Could you check a few things on this model? Use its own coordinates, in mm. A direction names the side the tool comes from. Round coordinates to 2 decimals unless told otherwise and drop trailing zeros. Write each loop counter-clockwise with the first axis right and the second up, starting at its lowest first coordinate (ties: lowest second). Pieces come first, ordered by that corner, then holes. Notation, with made-up numbers: (-0.75, -6) -> (31.25, -6) arc R13 ccw to (31.25, 18) -> close; hole circle Ø7 at (-17.75, -13). An arc over 180 degrees is marked (long way). One line per question, with ' | ' between items. Start each with the question number.
1. For faces 1 (the flat face through (-22.662, -5, 23)), 2 (the flat face through (4, 0, 1)), 3 (the flat face through (-17.224, -4.93, 22.376)), which set-ups out of +Z, -Z, +X, -X, +Y, -Y let a thin tool reach every point of the face, with its end or its side?
2. Imagine slicing it at C-C, the plane z = -1.5. List the corners of the cut face in (x, y) for me, and give its area (3 significant figures).
3. Thinking about a two-plate mould opening in Z: for faces 4 (the cylindrical face through (-0.357, -4.93, -12.358)), 5 (the flat face through (-16.59, -4.93, 24.41)), 6 (the flat face through (18.555, -4.93, 3.185)), which applies, released by +Z, released by -Z, zero draft, split by the parting line, or undercut?
4. If I drill on line 1 along X through (y, z) = (-0.5, 6); line 2 along Z through (x, y) = (-7.5, -1); line 3 along Z through (x, y) = (-16, -2), over which ranges is the centre line in solid material (lowest first)? Write a range as [from, to].
5. For pin 1 Ø6 at (x, y) = (12.5, -8.5) entering from +Z; pin 2 Ø3 at (x, y) = (6, -5) entering from +Z; pin 3 Ø6 at (y, z) = (-9, -17.5) entering from -X; pin 4 Ø8 at (x, z) = (19, 1) entering from -Y, each with a flat end and sliding along its axis, tell me the tip position at first contact or that it passes through.
6. Imagine slicing it at B-B, the plane y = -8. List the corners of the cut face in (x, z) for me.
7. Imagine slicing it at A-A, the plane x = -19. List the corners of the cut face in (y, z) for me, and give its area (3 significant figures).
8. Imagine slicing it at D-D, the plane z = 9. List the corners of the cut face in (x, y) for me, and give its area (3 significant figures).
from build123d import *

# Parameters (mm, degrees)
F0_R     = 3
F1_DEPTH = 10


with BuildPart() as f1:
    # F0 (on Front) → F1 (new body)
    with BuildSketch(Plane.XZ):
        with BuildLine():
            ThreePointArc((-11.631738, 22.991001), (-0.648629, -12.871174), (-37.288071, -20.888377))
            Line((-37.288071, -20.888377), (-38.549939, -22.690512))
            ThreePointArc((-38.549939, -22.690512), (-9.219197, -24.219506), (4.998539, 1.480421))
            ThreePointArc((4.998539, 1.480421), (7.215942, 5.906596), (12.154164, 6.255685))
            Line((12.154164, 6.255685), (25.138195, 0.026482))
            ThreePointArc((25.138195, 0.026482), (33.931194, -3.758973), (30.546238, 5.195834))
            Line((30.546238, 5.195834), (-10.680119, 24.974539))
            Line((-10.680119, 24.974539), (-22.661872, 23.830803))
            Line((-22.661872, 23.830803), (-22.661872, 21.77806))
            Line((-22.661872, 21.77806), (-11.631738, 22.991001))
        make_face()
        with Locations((30.338128, 0)):
            Circle(F0_R, mode=Mode.SUBTRACT)
    extrude(amount=F1_DEPTH)


solid = f1.part
Geometry results:
1) face 1: +Z, -X, +Y, -Y | face 2: +Z, -Z, +X, -X, +Y | face 3: +Y, -Y
2) outline: (2.79, -10) -> (5, -10) -> (5, 0) -> (2.79, 0) -> close; (25.36, -10) -> (27.74, -10) -> (27.74, 0) -> (25.36, 0) -> close; (32.94, -10) -> (35.32, -10) -> (35.32, 0) -> (32.94, 0) -> close | area: 69.7 mm2
3) face 4: undercut | face 5: released by +Z | face 6: released by -Z
4) line 1: x = [2.12, 7.36], [12.69, 28.87] | line 2: z = [-23.18, -20.5], [20.5, 23.45] | line 3: z = [-26.89, -24.61], [22.51, 24.47]
5) pin 1: stops at z = 15.29 | pin 2: stops at z = 17.69 | pin 3: stops at x = -7.5 | pin 4: stops at y = -10
6) outline: (-38.55, -22.69) arc R27.7 ccw to (5, 1.48) arc R5 cw to (12.15, 6.26) -> (25.14, 0.03) arc R5.2 ccw (long way) to (30.55, 5.2) -> (-10.68, 24.97) -> (-22.66, 23.83) -> (-22.66, 21.78) -> (-11.63, 22.99) arc R25.5 cw (long way) to (-37.29, -20.89) -> close; hole circle Ø6 at (30.34, 0)
7) outline: (-10, -27.46) -> (0, -27.46) -> (0, -25.24) -> (-10, -25.24) -> close; (-10, 22.18) -> (0, 22.18) -> (0, 24.18) -> (-10, 24.18) -> close | area: 42.2 mm2
8) outline: (1.2, -10) -> (22.62, -10) -> (22.62, 0) -> (1.2, 0) -> close | area: 214 mm2
